```python
from build123d import *

# Parameters (mm, degrees)
F1_DEPTH        = 2
F2_R            = 4.75
F3_DEPTH        = 20
F2_R_2          = 2.5
F4_DEPTH        = 2
F2_R_3          = 1.5
F5_DEPTH        = 25
F7_DEPTH        = 2
F8_D            = 5
F8_CSINK_D      = 8.5
F8_CSINK_ANGLE  = 90
F9_D            = 5
F9_CSINK_D      = 8.5
F9_CSINK_ANGLE  = 90
F10_D           = 5
F10_CSINK_D     = 8.5
F10_CSINK_ANGLE = 90


with BuildPart() as f1:
    # F0 (on Top) → F1 (new body)
    with BuildSketch(Plane.XY):
        with BuildLine():
            ThreePointArc((-57.5, -52.5), (-56.035534, -56.035534), (-52.5, -57.5))
            Line((-52.5, -57.5), (52.5, -57.5))
            ThreePointArc((52.5, -57.5), (56.035534, -56.035534), (57.5, -52.5))
            Line((57.5, -52.5), (57.5, 52.5))
            ThreePointArc((57.5, 52.5), (56.035534, 56.035534), (52.5, 57.5))
            Line((52.5, 57.5), (-52.5, 57.5))
            ThreePointArc((-52.5, 57.5), (-56.035534, 56.035534), (-57.5, 52.5))
            Line((-57.5, 52.5), (-57.5, -52.5))
        make_face()
    extrude(amount=F1_DEPTH)

    # F2 (on face) → F3 (join)
    with BuildSketch(Plane.XY.offset(2)):
        Circle(F2_R)
    extrude(amount=F3_DEPTH)

    # F2 (on face) → F4 (cut)
    with BuildSketch(Plane.XY.offset(2)):
        with Locations((47, -48)):
            Circle(F2_R_2)
        with Locations((0, 48)):
            Circle(F2_R_2)
        with Locations((-47, -48)):
            Circle(F2_R_2)
    extrude(amount=-F4_DEPTH, mode=Mode.SUBTRACT)

    # F2 (on face) → F5 (join)
    with BuildSketch(Plane.XY.offset(2)):
        with BuildLine():
            Line((-55.5, 49.5), (-55.5, 50.5))
            Line((-55.5, 50.5), (-51.5, 50.5))
            ThreePointArc((-51.5, 50.5), (-50.792893, 50.792893), (-50.5, 51.5))
            Line((-50.5, 51.5), (-50.5, 55.5))
            Line((-50.5, 55.5), (50.5, 55.5))
            Line((50.5, 55.5), (50.5, 51.5))
            ThreePointArc((50.5, 51.5), (50.792893, 50.792893), (51.5, 50.5))
            Line((51.5, 50.5), (55.5, 50.5))
            Line((55.5, 50.5), (55.5, -50.5))
            Line((55.5, -50.5), (51.5, -50.5))
            ThreePointArc((51.5, -50.5), (50.792893, -50.792893), (50.5, -51.5))
            Line((50.5, -51.5), (50.5, -55.5))
            Line((50.5, -55.5), (-50.5, -55.5))
            Line((-50.5, -55.5), (-50.5, -51.5))
            ThreePointArc((-50.5, -51.5), (-50.792893, -50.792893), (-51.5, -50.5))
            Line((-51.5, -50.5), (-55.5, -50.5))
            Line((-55.5, -50.5), (-55.5, 34.5))
            Line((-55.5, 34.5), (-57.5, 34.5))
            Line((-57.5, 34.5), (-57.5, -52.5))
            ThreePointArc((-57.5, -52.5), (-56.035534, -56.035534), (-52.5, -57.5))
            Line((-52.5, -57.5), (52.5, -57.5))
            ThreePointArc((52.5, -57.5), (56.035534, -56.035534), (57.5, -52.5))
            Line((57.5, -52.5), (57.5, 52.5))
            ThreePointArc((57.5, 52.5), (56.035534, 56.035534), (52.5, 57.5))
            Line((52.5, 57.5), (-52.5, 57.5))
            ThreePointArc((-52.5, 57.5), (-56.035534, 56.035534), (-57.5, 52.5))
            Line((-57.5, 52.5), (-57.5, 49.5))
            Line((-57.5, 49.5), (-55.5, 49.5))
        make_face()
        with Locations((-52.5, -52.5)):
            Circle(F2_R_3, mode=Mode.SUBTRACT)
        with Locations((52.5, -52.5)):
            Circle(F2_R_3, mode=Mode.SUBTRACT)
        with Locations((-52.5, 52.5)):
            Circle(F2_R_3, mode=Mode.SUBTRACT)
        with Locations((52.5, 52.5)):
            Circle(F2_R_3, mode=Mode.SUBTRACT)
    extrude(amount=F5_DEPTH)

    # F6 (on face) → F7 (join)
    with BuildSketch(Plane.XY.offset(27)):
        with BuildLine():
            Line((52.5, 57.5), (-52.5, 57.5))
            ThreePointArc((-52.5, 57.5), (-56.035534, 56.035534), (-57.5, 52.5))
            Line((-57.5, 52.5), (-57.5, 49.5))
            Line((-57.5, 49.5), (-56.5, 49.5))
            Line((-56.5, 49.5), (-56.5, 52.5))
            ThreePointArc((-56.5, 52.5), (-55.328427, 55.328427), (-52.5, 56.5))
            Line((-52.5, 56.5), (52.5, 56.5))
            ThreePointArc((52.5, 56.5), (55.328427, 55.328427), (56.5, 52.5))
            Line((56.5, 52.5), (56.5, -52.5))
            ThreePointArc((56.5, -52.5), (55.328427, -55.328427), (52.5, -56.5))
            Line((52.5, -56.5), (-52.5, -56.5))
            ThreePointArc((-52.5, -56.5), (-55.328427, -55.328427), (-56.5, -52.5))
            Line((-56.5, -52.5), (-56.5, 34.5))
            Line((-56.5, 34.5), (-57.5, 34.5))
            Line((-57.5, 34.5), (-57.5, -52.5))
            ThreePointArc((-57.5, -52.5), (-56.035534, -56.035534), (-52.5, -57.5))
            Line((-52.5, -57.5), (52.5, -57.5))
            ThreePointArc((52.5, -57.5), (56.035534, -56.035534), (57.5, -52.5))
            Line((57.5, -52.5), (57.5, 52.5))
            ThreePointArc((57.5, 52.5), (56.035534, 56.035534), (52.5, 57.5))
        make_face()
    extrude(amount=F7_DEPTH)

    # F8 (through all)
    with Locations(Plane.XY.offset(2)):
        with Locations((0, 48)):
            CounterSinkHole(F8_D / 2, F8_CSINK_D / 2, counter_sink_angle=F8_CSINK_ANGLE)

    # F9 (through all)
    with Locations(Plane.XY.offset(2)):
        with Locations((47, -48)):
            CounterSinkHole(F9_D / 2, F9_CSINK_D / 2, counter_sink_angle=F9_CSINK_ANGLE)

    # F10 (through all)
    with Locations(Plane.XY.offset(2)):
        with Locations((-47, -48)):
            CounterSinkHole(F10_D / 2, F10_CSINK_D / 2, counter_sink_angle=F10_CSINK_ANGLE)


solid = f1.part
```
Part model, mm, in its own coordinate system. A direction names the side the tool comes from. Round coordinates to 2 decimals unless told otherwise and drop trailing zeros. Write each loop counter-clockwise with the first axis right and the second up, starting at its lowest first coordinate (ties: lowest second). Pieces come first, ordered by that corner, then holes. Notation, with made-up numbers: (-18.5, 83) -> (16.5, 83) arc R23 cw to (16.5, 108) -> close; hole circle Ø1 at (33, -28.5). An arc over 180 degrees is marked (long way). Return JSON: item names as keys, results as strings. Group by question number.
Q1. Pin check, flat tips, straight feed: pin 1 (1.6 mm diameter, centred on x = -56.5, z = 21, fed in from +Y); pin 2 (12 mm diameter, centred on x = -40, y = 29, fed in from +Z); pin 3 (4.5 mm diameter, centred on y = 53, z = 20, fed in from -X); pin 4 (2.5 mm diameter, centred on x = -52.5, y = 52, fed in from +Z). Stop position of each tip, or through.
Q2. Saw through at A-A on x = 47. Write the cut outline in (y, z).
Q3. Probe L1, parallel to Y at x = -52.5, z = 20.75; L2, parallel to Y at x = -0.5, z = 6.25; L3, parallel to X at y = -48, z = 0.1. List the from-to ranges inside material, lowest first. Write a range as [from, to].
Q4. Mould opens along Y. For faces 3 (the cylindrical face through (51.3, 51.6, 14.3)), 4 (the flat face through (1, 57.5, 14)), 5 (the flat face through (-1, -57.5, 14)), 6 (the cylindrical face through (51.3, -53.4, 14.3)) say: pulls with the +Y half, pulls with the -Y half, needs draft (parallel to the pull), parting line crosses it, or undercut.
Q5. Saw through at C-C on y = -48. Write the cut outline in (x, z).
Q6. Which spindle directions (+Z, -Z, +X, -X, +Y, -Y) get a long thin tool onto all of the face, cutting with end or side? Do faces 1 (the flat face through (57.5, -1, 14)), 2 (the flat face through (53, 50.5, 14)). Say none if no direction does.
Q7. Saw through at B-B on z = 17.5. State how many separate pieces and enclosed holes the cut face has, plus the area to 3 significant figures.
Answer:
{
 "1": {"pin 1": "y = 56.34", "pin 2": "z = 2", "pin 3": "x = -57.5", "pin 4": "z = 27"},
 "2": {"outline": "(-57.5, 0) -> (-50.5, 0) -> (-50.5, 0.25) -> (-52.25, 2) -> (-55.5, 2) -> (-55.5, 27) -> (-56.5, 27) -> (-56.5, 29) -> (-57.5, 29) -> close; (-45.5, 0) -> (57.5, 0) -> (57.5, 29) -> (56.5, 29) -> (56.5, 27) -> (55.5, 27) -> (55.5, 2) -> (-43.75, 2) -> (-45.5, 0.25) -> close"},
 "3": {"L1": "[-57.5, -54], [-51, -50.5], [50.5, 51], [54, 57.5]", "L2": "[-57.5, -55.5], [-4.72, 4.72], [55.5, 57.5]", "L3": "[-57.5, -49.5], [-44.5, 44.5], [49.5, 57.5]"},
 "4": {"face 3": "undercut", "face 4": "pulls with the +Y half", "face 5": "pulls with the -Y half", "face 6": "undercut"},
 "5": {"outline": "(-57.5, 0) -> (-49.5, 0) -> (-49.5, 0.25) -> (-51.25, 2) -> (-55.5, 2) -> (-55.5, 27) -> (-56.5, 27) -> (-56.5, 29) -> (-57.5, 29) -> close; (-44.5, 0) -> (44.5, 0) -> (44.5, 0.25) -> (42.75, 2) -> (-42.75, 2) -> (-44.5, 0.25) -> close; (49.5, 0) -> (57.5, 0) -> (57.5, 29) -> (56.5, 29) -> (56.5, 27) -> (55.5, 27) -> (55.5, 2) -> (51.25, 2) -> (49.5, 0.25) -> close"},
 "6": {"face 1": "+Z, -Z, +X, +Y, -Y", "face 2": "+Z"},
 "7": {"separate pieces": "2", "enclosed holes": "4", "area": "994 mm2"}
}
